Input: part model. Units: mm. Frame: model coordinates. Face numbers are marked on the shaded views. Give positions to 0.01 mm unless a question says otherwise; leave off trailing zeros. Loops run counter-clockwise (first coordinate to the right, second up) from the corner with the lowest first, then second, coordinate; pieces in that order, holes last. Notation, with made-up numbers: (-15, 52.25) -> (38, 52.25) arc R10 ccw to (38, 56.25) -> close; hole circle Ø10 at (-24.75, 27.25). An arc over 180 degrees is marked (long way). Answer as a JSON object with one key per item and string values.
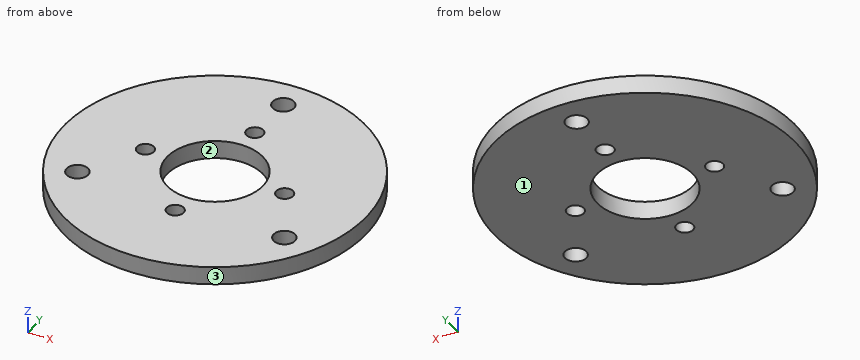
```python
from build123d import *

# Parameters (mm, degrees)
SKETCH1_R                    = 15.875
SKETCH1_R_2                  = 3.96875
BOSS_EXTRUDE1_DEPTH          = 1.905
X_0_397_DIAMETER_HOLE1_D     = 10.0838
X_0_397_DIAMETER_HOLE1_DEPTH = 12.7
X_0_397_DIAMETER_HOLE1_TIP   = 3.029479155
CIRPATTERN1_COUNT            = 3
CIRPATTERN2_COUNT            = 4


with BuildPart() as part:
    # Sketch1 → Boss-Extrude1 (new body)
    with BuildSketch(Plane.XY):
        with Locations(Location((0, 0, 0), (0, 0, 180))):
            Circle(SKETCH1_R)
        with Locations(Location((0, 0, 0), (0, 0, 180))):
            Circle(SKETCH1_R_2, mode=Mode.SUBTRACT)
    extrude(amount=BOSS_EXTRUDE1_DEPTH)

    # X (0.397) Diameter Hole1
    with Locations(Plane.XY.offset(1.905)):
        with Locations((0, 0)):
            Hole(X_0_397_DIAMETER_HOLE1_D / 2, depth=X_0_397_DIAMETER_HOLE1_DEPTH)
            with Locations((0, 0, -(X_0_397_DIAMETER_HOLE1_DEPTH + X_0_397_DIAMETER_HOLE1_TIP / 2))):  # 118° drill point
                Cone(0, X_0_397_DIAMETER_HOLE1_D / 2, X_0_397_DIAMETER_HOLE1_TIP, mode=Mode.SUBTRACT)

    # Sketch4 → #4-40 Tapped Hole1 (revolve, cut)
    with BuildSketch(Plane(origin=(0, 12.7, 1.905), x_dir=(0, -1, 0), z_dir=(1, 0, 0))):
        Polygon((0, 0), (0, 9.543752758), (1.1303, 8.8646), (1.1303, 0), align=None)
    f_4_40_tapped_hole1 = revolve(axis=Axis((0, 12.7, 8.255), (0, 0, -1)), mode=Mode.SUBTRACT)

    # CirPattern1: #4-40 Tapped Hole1 ×3 about axis
    cirpattern1_axis = Axis((0, 0, 0), (0, 0, 1))
    for i in range(1, CIRPATTERN1_COUNT):
        add(f_4_40_tapped_hole1.rotate(cirpattern1_axis, i * 360 / CIRPATTERN1_COUNT), mode=Mode.SUBTRACT)

    # Sketch6 → #2-56 Tapped Hole1 (revolve, cut)
    with BuildSketch(Plane(origin=(0, 7.4, 1.905), x_dir=(0, -1, 0), z_dir=(1, 0, 0))):
        Polygon((0, 0), (0, 7.18896509), (0.889, 6.6548), (0.889, 0), align=None)
    f_2_56_tapped_hole1 = revolve(axis=Axis((0, 7.4, 8.255), (0, 0, -1)), mode=Mode.SUBTRACT)

    # CirPattern2: #2-56 Tapped Hole1 ×4 about axis
    cirpattern2_axis = Axis((0, 0, 0), (0, 0, 1))
    for i in range(1, CIRPATTERN2_COUNT):
        add(f_2_56_tapped_hole1.rotate(cirpattern2_axis, i * 360 / CIRPATTERN2_COUNT), mode=Mode.SUBTRACT)


solid = part.part
```
Q1. Draft query along Y for the marked faces 1, 2 and 3. Return one class per face: +Y half, -Y half, draft (parallel to the pull), parting line (faces both ways), or undercut.
Evaluation:
{"face 1": "draft", "face 2": "undercut", "face 3": "parting line"}
Q2. Pin query (flat end, axial travel): pin 1 (9 mm diameter, centred on x = 0, y = 0, fed in from +Z). Return the tip coordinate at first contact, or that it passes through.
Evaluation:
{"pin 1": "passes through"}
Q3. Section D-D, the plane x = -4. Return the cut outline in (y, z) (3 decimals), then the cut area to 3 significant figures.
Evaluation:
{"outline": "(-15.363, 0) -> (-3.069, 0) -> (-3.069, 1.905) -> (-15.363, 1.905) -> close; (3.069, 0) -> (15.363, 0) -> (15.363, 1.905) -> (3.069, 1.905) -> close", "area": "46.8 mm2"}
Q4. Ray query, line 1 along Y through (x, z) = (0, 1.3) (3 decimals); line 2 along X through (y, z) = (-7, 1.8); line 3 along X through (y, z) = (-5.5, 0.25). Return the intervals inside material, ascending.
Evaluation:
{"line 1": "y = -15.875 to -8.289, -6.511 to -5.042, 5.042 to 6.511, 8.289 to 11.57, 13.83 to 15.875", "line 2": "x = -14.25 to -11.92, -10.07 to -0.79, 0.79 to 10.07, 11.92 to 14.25", "line 3": "x = -14.89 to -11.74, -10.25 to 10.25, 11.74 to 14.89"}
Q5. Section A-A, the plane x = 0. Return the cut outline in (y, z) (3 decimals), then the cut area to 3 significant figures.
Evaluation:
{"outline": "(-15.875, 0) -> (-8.289, 0) -> (-8.289, 1.905) -> (-15.875, 1.905) -> close; (-6.511, 0) -> (-5.042, 0) -> (-5.042, 1.905) -> (-6.511, 1.905) -> close; (5.042, 0) -> (6.511, 0) -> (6.511, 1.905) -> (5.042, 1.905) -> close; (8.289, 0) -> (11.57, 0) -> (11.57, 1.905) -> (8.289, 1.905) -> close; (13.83, 0) -> (15.875, 0) -> (15.875, 1.905) -> (13.83, 1.905) -> close", "area": "30.2 mm2"}
Q6. Section C-C, the plane y = -4.5. Return the cut outline in (x, z) (3 decimals).
Evaluation:
{"outline": "(-15.224, 0) -> (-2.274, 0) -> (-2.274, 1.905) -> (-15.224, 1.905) -> close; (2.274, 0) -> (15.224, 0) -> (15.224, 1.905) -> (2.274, 1.905) -> close"}
Q7. Section B-B, the plane y = 0. Return the cut outline in (x, z) (3 decimals).
Evaluation:
{"outline": "(-15.875, 0) -> (-8.289, 0) -> (-8.289, 1.905) -> (-15.875, 1.905) -> close; (-6.511, 0) -> (-5.042, 0) -> (-5.042, 1.905) -> (-6.511, 1.905) -> close; (5.042, 0) -> (6.511, 0) -> (6.511, 1.905) -> (5.042, 1.905) -> close; (8.289, 0) -> (15.875, 0) -> (15.875, 1.905) -> (8.289, 1.905) -> close"}
